Part model, mm, in its own coordinate system. A direction names the side the tool comes from. Give positions to 0.01 mm unless a question says otherwise; leave off trailing zeros. Write each loop counter-clockwise with the first axis right and the second up, starting at its lowest first coordinate (ties: lowest second). Pieces come first, ordered by that corner, then holes. Notation, with made-up numbers: (-39, 49) - (-23, 49) arc R8 ccw to (-23, 54) - close; hole circle Ø5 at (31, -25). An arc over 180 degrees is marked (long way). Answer as a JSON object with one key per item and string values. Group by question number.
```python
from build123d import *

# Parameters (mm, degrees)
SKETCH1_W           = 85
SKETCH1_H           = 35
BOSS_EXTRUDE1_DEPTH = 20
SHELL1_T            = -3
SKETCH3_W           = 17
SKETCH3_H           = 15
CUT_EXTRUDE1_DEPTH  = 20
SKETCH4_W           = 73
SKETCH4_H           = 25
CUT_EXTRUDE2_DEPTH  = 20


with BuildPart() as part:
    # Sketch1 → Boss-Extrude1 (new body)
    with BuildSketch(Plane.XY):
        Rectangle(SKETCH1_W, SKETCH1_H)
    extrude(amount=BOSS_EXTRUDE1_DEPTH)

    # Shell1
    shell1_openings = [part.faces().sort_by_distance(p)[0] for p in [
        (0, 0, 0),
    ]]
    offset(amount=SHELL1_T, openings=shell1_openings, kind=Kind.INTERSECTION)

    # Sketch3 → Cut-Extrude1 (cut)
    with BuildSketch(Plane.ZY.offset(42.5)):
        with Locations((8.5, 0)):
            Rectangle(SKETCH3_W, SKETCH3_H)
    extrude(amount=-CUT_EXTRUDE1_DEPTH, mode=Mode.SUBTRACT)

    # Sketch4 → Cut-Extrude2 (cut)
    with BuildSketch(Plane.XY.offset(20)):
        Rectangle(SKETCH4_W, SKETCH4_H)
    extrude(amount=-CUT_EXTRUDE2_DEPTH, mode=Mode.SUBTRACT)


solid = part.part
```
1) Band-saw the part on B-B (x = -18). List the corners of the cut face in (y, z).
2) Band-saw the part on C-C (z = 18.25). List the corners of the cut face in (x, y).
3) Band-saw the part on A-A (y = 9.5). List the corners of the cut face in (x, z).
4) Probe line 1 (Y direction, x = 29, z = 14.5); line 2 (X direction, y = 1.5, z = 18.25); line 3 (X direction, y = -13.5, z = 10). List the from-to ranges inside material, lowest first.
5) Drop flat-ended pins along their axis: P1, Ø1.5, axis at x = 17.5, y = 11.5, coming from the -Z side; P2, Ø6, axis at x = 18, y = 14, coming from the -Z side; P3, Ø3, axis at y = -1.5, z = 9, coming from the -X side. Give the stop position or say it passes through.
6) Band-saw the part on D-D (y = 3). List the corners of the cut face in (x, z), plus the area to 3 significant figures.
7) Which spindle directions (+Z, -Z, +X, -X, +Y, -Y) get a long thin tool onto all of the face, cutting with end or side? Do faces 1 (the flat face through (42.5, 0, 10)), 2 (the flat face through (-41, -7.5, 8)), 3 (the flat face through (36.5, 0, 19)), 4 (the flat face through (-1, -14.5, 8)), 5 (the flat face through (-1, -17.5, 10)). Say none if no direction does.
8) Mould opens along Y. For faces 6 (the flat face through (39.5, 0, 8)), 7 (the flat face through (-1, 17.5, 10)), 8 (the flat face through (-1, -15, 20)) say: pulls with the +Y half, pulls with the -Y half, needs draft (parallel to the pull), parting line crosses it, or undercut.
Verdict:
{
 "1": {"outline": "(-17.5, 0) - (-14.5, 0) - (-14.5, 17) - (-12.5, 17) - (-12.5, 20) - (-17.5, 20) - close; (12.5, 17) - (14.5, 17) - (14.5, 0) - (17.5, 0) - (17.5, 20) - (12.5, 20) - close"},
 "2": {"outline": "(-42.5, -17.5) - (42.5, -17.5) - (42.5, 17.5) - (-42.5, 17.5) - close; hole (-36.5, -12.5) - (36.5, -12.5) - (36.5, 12.5) - (-36.5, 12.5) - close"},
 "3": {"outline": "(-42.5, 0) - (-39.5, 0) - (-39.5, 17) - (-36.5, 17) - (-36.5, 20) - (-42.5, 20) - close; (36.5, 17) - (39.5, 17) - (39.5, 0) - (42.5, 0) - (42.5, 20) - (36.5, 20) - close"},
 "4": {"line 1": "-17.5 to -14.5, 14.5 to 17.5", "line 2": "-42.5 to -36.5, 36.5 to 42.5", "line 3": "-42.5 to -39.5, 39.5 to 42.5"},
 "5": {"P1": "through", "P2": "z = 0", "P3": "x = 39.5"},
 "6": {"outline": "(-42.5, 17) - (-36.5, 17) - (-36.5, 20) - (-42.5, 20) - close; (36.5, 17) - (39.5, 17) - (39.5, 0) - (42.5, 0) - (42.5, 20) - (36.5, 20) - close", "area": "87.0 mm2"},
 "7": {"face 1": "+Z, -Z, +X, +Y, -Y", "face 2": "-Z, -X", "face 3": "+Z, -Z", "face 4": "-Z", "face 5": "+Z, -Z, +X, -X, -Y"},
 "8": {"face 6": "undercut", "face 7": "pulls with the +Y half", "face 8": "needs draft"}
}
